from build123d import *

# Parameters (mm, degrees)
SKETCH1_R               = 3.75
BOSS_EXTRUDE1_DEPTH     = 0.88
SKETCH2_R               = 2.125
BOSS_EXTRUDE2_DEPTH     = 1.12
SKETCH3_R               = 2.5
BOSS_EXTRUDE3_DEPTH     = 0.0625
SKETCH4_R               = 1.785
CUT_EXTRUDE1_DEPTH      = 3
CUT_EXTRUDE1_DEPTH_BACK = 1.0625
SKETCH7_R               = 0.375
CUT_EXTRUDE2_DEPTH      = 3.0625
CIRPATTERN1_COUNT       = 4
SCALE1_SCALE            = 25.4


with BuildPart() as part:
    # Sketch1 → Boss-Extrude1 (new body)
    with BuildSketch(Plane(origin=(0, 0, 0), x_dir=(1, 0, 0), z_dir=(0, 1, 0))):
        Circle(SKETCH1_R)
    extrude(amount=BOSS_EXTRUDE1_DEPTH)

    # Sketch2 → Boss-Extrude2 (add)
    with BuildSketch(Plane(origin=(0, 0, 0), x_dir=(1, 0, 0), z_dir=(0, 1, 0))):
        Circle(SKETCH2_R)
    extrude(amount=BOSS_EXTRUDE2_DEPTH)

    # Sketch3 → Boss-Extrude3 (add)
    with BuildSketch(Plane(origin=(0, 0, 0), x_dir=(1, 0, 0), z_dir=(0, 1, 0))):
        Circle(SKETCH3_R)
    extrude(amount=-BOSS_EXTRUDE3_DEPTH)

    # Sketch4 → Cut-Extrude1 (cut, two sides)
    with BuildSketch(Plane(origin=(0, 0, 0), x_dir=(1, 0, 0), z_dir=(0, 1, 0))) as cut_extrude1_sk:
        Circle(SKETCH4_R)
    extrude(amount=CUT_EXTRUDE1_DEPTH, mode=Mode.SUBTRACT)
    extrude(cut_extrude1_sk.sketch, amount=-CUT_EXTRUDE1_DEPTH_BACK, mode=Mode.SUBTRACT)

    # Sketch7 → Cut-Extrude2 (cut)
    with BuildSketch(Plane(origin=(0, 0, 0), x_dir=(1, 0, 0), z_dir=(0, 1, 0))):
        with Locations((0, 3)):
            Circle(SKETCH7_R)
    cut_extrude2 = extrude(amount=CUT_EXTRUDE2_DEPTH, mode=Mode.SUBTRACT)

    # CirPattern1: Cut-Extrude2 ×4 about axis
    cirpattern1_axis = Axis((0, 0, 0), (0, 1, 0))
    for i in range(1, CIRPATTERN1_COUNT):
        add(cut_extrude2.rotate(cirpattern1_axis, i * 360 / CIRPATTERN1_COUNT), mode=Mode.SUBTRACT)


with BuildPart() as part_1:
    # Scale1: scaled about (0, 0.449224649, 0)
    add(part.part.scale(SCALE1_SCALE).moved(Location((0, -10.961081436, 0))))


solid = part_1.part
Could you check a few things on this model? Use its own coordinates, in mm. A direction names the side the tool comes from. Round coordinates to 2 decimals unless told otherwise and drop trailing zeros. Write each loop counter-clockwise with the first axis right and the second up, starting at its lowest first coordinate (ties: lowest second). Pieces come first, ordered by that corner, then holes. Notation, with made-up numbers: (57, 31) -> (100, 31) arc R19 cw to (100, 63) -> close; hole circle Ø10 at (49, 54.5). An arc over 180 degrees is marked (long way). Use a Markdown table: item, result.
1. If we section it at A-A (x = 76.2): List the corners of the cut face in (y, z) for me (3 decimals), then the cut area to 3 significant figures.
Answer key:
| item | result |
|---|---|
| outline | (-10.961, -57.15) -> (11.391, -57.15) -> (11.391, -9.525) -> (-10.961, -9.525) -> close; (-10.961, 9.525) -> (11.391, 9.525) -> (11.391, 57.15) -> (-10.961, 57.15) -> close |
| area | 2,130 mm^2 |
2. We'd pull the mould along X, two halves only. Please class faces 4 (the face through (-35.98, 2.68, 27.59)), 5 (the face through (-13.77, -11.74, 61.99)), 6 (the face through (-15, -12.549, -43)): +X half, -X half, draft (parallel to the pull), parting line (faces both ways), or undercut.
Answer key:
| item | result |
|---|---|
| face 4 | undercut |
| face 5 | parting line |
| face 6 | draft |
3. For pin 1 Ø15 at (x, z) = (0, 76.2) entering from +Y; pin 2 Ø10 at (y, z) = (4.5, -3) entering from +X; pin 3 Ø2 at (x, y) = (40, 13) entering from -Z; pin 4 Ø22 at (x, z) = (0, -76.2) entering from -Y, each with a flat end and sliding along its axis, tell me the tip position at first contact or that it passes through.
Answer key:
| item | result |
|---|---|
| pin 1 | passes through |
| pin 2 | stops at x = 95.25 |
| pin 3 | stops at z = -37.31 |
| pin 4 | stops at y = -10.96 |
4. If we section it at C-C (y = -8): List the corners of the cut face in (x, z) for me (3 decimals).
Answer key:
| item | result |
|---|---|
| outline | circle Ø190.5 at (0, 0); hole circle Ø19.05 at (-76.2, 0); hole circle Ø90.678 at (0, 0); hole circle Ø19.05 at (0, -76.2); hole circle Ø19.05 at (0, 76.2); hole circle Ø19.05 at (76.2, 0) |
5. If we section it at D-D (z = 0): List the corners of the cut face in (x, y) for me (3 decimals).
Answer key:
| item | result |
|---|---|
| outline | (-95.25, -10.961) -> (-85.725, -10.961) -> (-85.725, 11.391) -> (-95.25, 11.391) -> close; (-66.675, -10.961) -> (-63.5, -10.961) -> (-63.5, -12.549) -> (-45.339, -12.549) -> (-45.339, 17.487) -> (-53.975, 17.487) -> (-53.975, 11.391) -> (-66.675, 11.391) -> close; (45.339, -12.549) -> (63.5, -12.549) -> (63.5, -10.961) -> (66.675, -10.961) -> (66.675, 11.391) -> (53.975, 11.391) -> (53.975, 17.487) -> (45.339, 17.487) -> close; (85.725, -10.961) -> (95.25, -10.961) -> (95.25, 11.391) -> (85.725, 11.391) -> close |
6. If we section it at B-B (z = -76.2): List the corners of the cut face in (x, y) for me (3 decimals), then the cut area to 3 significant figures.
Answer key:
| item | result |
|---|---|
| outline | (-57.15, -10.961) -> (-9.525, -10.961) -> (-9.525, 11.391) -> (-57.15, 11.391) -> close; (9.525, -10.961) -> (57.15, -10.961) -> (57.15, 11.391) -> (9.525, 11.391) -> close |
| area | 2,130 mm^2 |
7. Which directions (+Z, -Z, +X, -X, +Y, -Y) give clear straight access to the entire face, cutting with the end or side of a thin tool? Please do faces 1 (the face through (-2.06, 0.06, -66.9)), 2 (the face through (-1, -10.961, -65)), 3 (the face through (29.02, 14.4, -45.51)).
Answer key:
| item | result |
|---|---|
| face 1 | +Y, -Y |
| face 2 | -Y |
| face 3 | +Y |
8. Please list where these lines run through material, in increasing order: probe 1 along X at (y, z) = (6.5, 0) (3 decimals); probe 2 along X at (y, z) = (5, -4).
Answer key:
| item | result |
|---|---|
| probe 1 | x = -95.25 to -85.725, -66.675 to -45.339, 45.339 to 66.675, 85.725 to 95.25 |
| probe 2 | x = -95.17 to -84.84, -67.56 to -45.16, 45.16 to 67.56, 84.84 to 95.17 |
